```python
from build123d import *

# Parameters (mm, degrees)
BOSS_EXTRUDE1_DEPTH                  = 194.071875
F_10_32_TAPPED_HOLE1_D               = 4.0386
F_10_32_TAPPED_HOLE1_DEPTH           = 16.34744
F_10_32_TAPPED_HOLE1_TIP             = 1.213317848
F_10_32_TAPPED_HOLE1_ON_FACE_2_D     = 4.0386
F_10_32_TAPPED_HOLE1_ON_FACE_2_DEPTH = 16.34744
F_10_32_TAPPED_HOLE1_ON_FACE_2_TIP   = 1.213317848


with BuildPart() as part:
    # Sketch1 → Boss-Extrude1 (new, symmetric)
    with BuildSketch(Plane(origin=(0, 0, 0), x_dir=(0, 0, -1), z_dir=(1, 0, 0))):
        Polygon((0, 7.332348419), (-6.35, 3.666174209), (-6.35, -3.666174209), (0, -7.332348419), (6.35, -3.666174209), (6.35, 3.666174209), align=None)
    extrude(amount=BOSS_EXTRUDE1_DEPTH, both=True)

    # #10-32 Tapped Hole1
    with Locations(Plane(origin=(194.071875, 0, 0), x_dir=(0, 0, 1), z_dir=(1, 0, 0))):
        with Locations((0, 0)):
            Hole(F_10_32_TAPPED_HOLE1_D / 2, depth=F_10_32_TAPPED_HOLE1_DEPTH)
            with Locations((0, 0, -(F_10_32_TAPPED_HOLE1_DEPTH + F_10_32_TAPPED_HOLE1_TIP / 2))):  # 118° drill point
                Cone(0, F_10_32_TAPPED_HOLE1_D / 2, F_10_32_TAPPED_HOLE1_TIP, mode=Mode.SUBTRACT)

    # #10-32 Tapped Hole1 on face 2
    with Locations(Plane(origin=(-194.071875, 0, 0), x_dir=(0, 0, -1), z_dir=(-1, 0, 0))):
        with Locations((0, 0)):
            Hole(F_10_32_TAPPED_HOLE1_ON_FACE_2_D / 2, depth=F_10_32_TAPPED_HOLE1_ON_FACE_2_DEPTH)
            with Locations((0, 0, -(F_10_32_TAPPED_HOLE1_ON_FACE_2_DEPTH + F_10_32_TAPPED_HOLE1_ON_FACE_2_TIP / 2))):  # 118° drill point
                Cone(0, F_10_32_TAPPED_HOLE1_ON_FACE_2_D / 2, F_10_32_TAPPED_HOLE1_ON_FACE_2_TIP, mode=Mode.SUBTRACT)


solid = part.part
```
Verification items for the finished model (mm, model axes). Round coordinates to 2 decimals unless told otherwise and drop trailing zeros. Write each loop counter-clockwise with the first axis right and the second up, starting at its lowest first coordinate (ties: lowest second). Pieces come first, ordered by that corner, then holes. Notation, with made-up numbers: (8, 85) -> (51, 85) arc R33 ccw to (51, 117) -> close; hole circle Ø6 at (71, -9). An arc over 180 degrees is marked (long way). Write each question's results on one line, items separated by ' | '. Start each with the question number.
1. Cross-section at B-B (z = 4.25). Enter the section's corners in (x, y), then the cut area to 3 significant figures.
2. Depth check by flat-ended pin: P1, Ø1.5, axis at x = 152, z = -4, coming from the -Y side; P2, Ø2.5, axis at y = 0, z = 0, coming from the -X side; P3, Ø3, axis at x = -23, z = 2.5, coming from the +Y side (3 decimals). Enter the tip coordinate at first touch or a pass-through.
3. Cross-section at A-A (x = 133.5). Enter the section's corners in (y, z), then the cut area to 3 significant figures.
4. Material ranges on probe 1 along Y at (x, z) = (183, 0); probe 2 along Y at (x, z) = (-162.5, -1.75); probe 3 along X at (y, z) = (-0.5, -0.25), recorded low to high. Write a range as from..to.
Solutions:
1) outline: (-194.07, -4.88) -> (194.07, -4.88) -> (194.07, 4.88) -> (-194.07, 4.88) -> close | area: 3,790 mm2
2) P1: stops at y = -5.46 | P2: stops at x = -177.26 | P3: stops at y = 6.755
3) outline: (-7.33, 0) -> (-3.67, -6.35) -> (3.67, -6.35) -> (7.33, 0) -> (3.67, 6.35) -> (-3.67, 6.35) -> close | area: 140 mm2
4) probe 1: y = -7.33..-2.02, 2.02..7.33 | probe 2: y = -6.32..6.32 | probe 3: x = -176.85..176.85
